from build123d import *

# Parameters (mm, degrees)
F0_R     = 1
F1_DEPTH = 4


with BuildPart() as f1:
    # F0 (on Front) → F1 (new body)
    with BuildSketch(Plane.XZ):
        with BuildLine():
            ThreePointArc((0, -2), (1.414214, -1.414214), (2, 0))
            ThreePointArc((2, 0), (1.414214, 1.414214), (0, 2))
            ThreePointArc((0, 2), (-1.414197, 1.41423), (-2, 4.6e-05))
            ThreePointArc((-2, 4.6e-05), (-1.41423, -1.414197), (0, -2))
        make_face()
        Circle(F0_R, mode=Mode.SUBTRACT)
        with BuildLine():
            Line((2, -1.535898), (2, 0))
            ThreePointArc((2, 0), (1.414214, -1.414214), (0, -2))
            Line((0, -2), (0, -9))
            Line((0, -9), (2, -1.535898))
        make_face()
        with BuildLine():
            ThreePointArc((-2, 4.6e-05), (-1.414197, 1.41423), (0, 2))
            Line((0, 2), (-6, 2))
            Line((-6, 2), (-6, 4.095806))
            Line((-6, 4.095806), (-7.433941, 2.047926))
            Line((-7.433941, 2.047926), (-6, 4.6e-05))
            Line((-6, 4.6e-05), (-2, 4.6e-05))
        make_face()
    extrude(amount=F1_DEPTH)


solid = f1.part
For this review, take the finished solid that the model builds, in its own axes (mm). A direction names the side the tool comes from. Round coordinates to 2 decimals unless told otherwise and drop trailing zeros. Loops run counter-clockwise (first coordinate to the right, second up) from the corner with the lowest first, then second, coordinate; pieces in that order, holes last. Notation, with made-up numbers: (-11, -26) - (26, -26) arc R18 ccw to (26, 9) - close; hole circle Ø7 at (77, -15). An arc over 180 degrees is marked (long way). Use one line per item in the form item = value.
1) We need section D-D on x = -2.5. Write out the cut boundary in (y, z).
Solutions:
outline = (-4, 0) - (0, 0) - (0, 2) - (-4, 2) - close
2) Tool access review of faces 1 (the face through (-4, -2, 0)), 2 (the face through (-6, -2, 3)), 3 (the face through (2, -2, -1)): name each direction out of +Z, -Z, +X, -X, +Y, -Y from which nothing blocks a thin tool from reaching the whole face with its end or side.
Solutions:
face_1 = -Z, -X, +Y, -Y
face_2 = +Z, +X, +Y, -Y
face_3 = +Z, -Z, +X, +Y, -Y
3) Wall thickness on probe 1 along Z at (x, y) = (-4, -3.4); probe 2 along X at (y, z) = (-1.05, 0.5); probe 3 along X at (y, z) = (-1.8, -0.25): over which ranges is each line inside the solid? List them lowest first.
Solutions:
probe_1 = 0 to 2
probe_2 = -6.35 to -0.87, 0.87 to 1.94
probe_3 = -1.98 to -0.97, 0.97 to 2
4) We need section A-A on y = -1. Write out the cut boundary in (x, z).
Solutions:
outline = (-7.43, 2.05) - (-6, 0) - (-2, 0) arc R2 ccw to (0, -2) - (0, -9) - (2, -1.54) - (2, 0) arc R2 ccw to (0, 2) - (-6, 2) - (-6, 4.1) - close; hole circle Ø2 at (0, 0)
5) We need section B-B on z = 0.75. Write out the cut boundary in (x, y).
Solutions:
outline = (-6.53, -4) - (-0.66, -4) - (-0.66, 0) - (-6.53, 0) - close; (0.66, -4) - (1.85, -4) - (1.85, 0) - (0.66, 0) - close
6) We need section C-C on x = 0.5. Write out the cut boundary in (y, z).
Solutions:
outline = (-4, -7.13) - (0, -7.13) - (0, -0.87) - (-4, -0.87) - close; (-4, 0.87) - (0, 0.87) - (0, 1.94) - (-4, 1.94) - close
7) Clearance check with flat-ended pins moving along their axes: P1, Ø1.7, axis at y = -3, z = 3.5, coming from the +X side; P2, Ø1.6, axis at x = 0, z = 0, coming from the +Y side; P3, Ø2, axis at y = -2.5, z = -7.5, coming from the -X side. State where each tip first meets the part, or that it passes through.
Solutions:
P1 = -6
P2 = through
P3 = 0
8) Mouldability with a two-part tool opening along X and no side actions: class faces 4 (the face through (-6.707, -1.972, 3.086)), 5 (the face through (0, -2, -1)), 6 (the face through (1.43, -1.97, 1.4)), 7 (the face through (-1.7, -4, -0.5)) as pulls with the +X half, pulls with the -X half, needs draft (parallel to the pull), parting line crosses it, or undercut.
Solutions:
face_4 = pulls with the -X half
face_5 = undercut
face_6 = pulls with the +X half
face_7 = needs draft
